```python
from build123d import *

# Parameters (mm, degrees)
F1_DEPTH = 2
F2_R     = 0.5
F3_R     = 2
F4_SIZE  = 0.49999


# Not quite as in the source:
# - a fillet or chamfer is up to 0.001 mm smaller than in the source, because OpenCascade refuses the exact size


with BuildPart() as f1:
    # F0 (on Top) → F1 (new body)
    with BuildSketch(Plane.XY):
        Polygon((-14.4337567297, 0), (-7.2168783649, 12.5), (7.2168783649, 12.5), (9.5262794416, 12.5), (10.68097998, 12.5), (17.8978583449, 0), (8.9489291724, -15.5), (-8.9489291724, -15.5), (-17.8978583449, 0), (-8.9489291724, 15.5), (8.9489291724, 15.5), (10.1036297108, 17.5), (-10.1036297108, 17.5), (-20.2072594216, 0), (-10.1036297108, -17.5), (10.1036297108, -17.5), (20.2072594216, 0), (11.8356805184, 14.5), (8.3715789032, 14.5), (-8.3715789032, 14.5), (-16.7431578065, 0), (-8.3715789032, -14.5), (8.3715789032, -14.5), (16.7431578065, 0), (14.4337567297, 0), (7.2168783649, -12.5), (-7.2168783649, -12.5), align=None)
    extrude(amount=F1_DEPTH)

    # F2
    f2_edges = [f1.edges().sort_by_distance(p)[0] for p in [
        (16.743158, 0, 1),
        (14.433757, 0, 1),
        (10.10363, 17.5, 1),
        (8.948929, 15.5, 1),
    ]]
    fillet(f2_edges, radius=F2_R)

    # F3
    f3_edges = [f1.edges().sort_by_distance(p)[0] for p in [
        (-10.10363, 17.5, 1),
        (-20.207259, 0, 1),
        (-10.10363, -17.5, 1),
        (10.10363, -17.5, 1),
        (20.207259, 0, 1),
        (11.835681, 14.5, 1),
        (-8.371579, 14.5, 1),
        (-16.743158, 0, 1),
        (-8.371579, -14.5, 1),
        (8.371579, -14.5, 1),
    ]]
    fillet(f3_edges, radius=F3_R)

    # F4 (size 0.5 in the source; OpenCascade refuses exactly that, so slightly less here)
    f4_edges = [f1.edges().sort_by_distance(p)[0] for p in [
        (12.629537, -7.125, 0),
        (8.216878, -14.232051, 0),
        (16.310145, -0.25, 0),
        (0, -14.5, 0),
        (15.299782, 0, 0),
        (-8.216878, -14.232051, 0),
        (14.472432, -0.066987, 0),
        (-12.557368, -7.25, 0),
        (10.753149, -6.375, 0),
        (-16.433757, 0, 0),
        (0, -12.5, 0),
        (-12.557368, 7.25, 0),
        (-10.825318, -6.25, 0),
        (-8.216878, 14.232051, 0),
        (-10.825318, 6.25, 0),
        (1.732051, 14.5, 0),
        (1.732051, 12.5, 0),
        (11.68098, 14.232051, 0),
        (14.289419, 6.25, 0),
        (16.02147, 7.25, 0),
        (13.423394, -7.75, 0),
        (19.897858, 0, 0),
        (0, -15.5, 0),
        (15.155445, -8.75, 0),
        (-13.423394, -7.75, 0),
        (9.948929, -17.232051, 0),
        (-13.423394, 7.75, 0),
        (0, -17.5, 0),
        (-0.144338, 15.5, 0),
        (-9.948929, -17.232051, 0),
        (8.910254, 15.566987, 0),
        (-15.155445, -8.75, 0),
        (9.381942, 16.25, 0),
        (-19.897858, 0, 0),
        (9.670617, 17.25, 0),
        (-15.155445, 8.75, 0),
        (0.144338, 17.5, 0),
        (-9.948929, 17.232051, 0),
        (12.629537, -7.125, 2),
        (8.216878, -14.232051, 2),
        (16.310145, -0.25, 2),
        (0, -14.5, 2),
        (15.299782, 0, 2),
        (-8.216878, -14.232051, 2),
        (14.472432, -0.066987, 2),
        (-12.557368, -7.25, 2),
        (10.753149, -6.375, 2),
        (-16.433757, 0, 2),
        (0, -12.5, 2),
        (-12.557368, 7.25, 2),
        (-10.825318, -6.25, 2),
        (-8.216878, 14.232051, 2),
        (-10.825318, 6.25, 2),
        (1.732051, 14.5, 2),
        (1.732051, 12.5, 2),
        (11.68098, 14.232051, 2),
        (14.289419, 6.25, 2),
        (16.02147, 7.25, 2),
        (13.423394, -7.75, 2),
        (19.897858, 0, 2),
        (0, -15.5, 2),
        (15.155445, -8.75, 2),
        (-13.423394, -7.75, 2),
        (9.948929, -17.232051, 2),
        (-13.423394, 7.75, 2),
        (0, -17.5, 2),
        (-0.144338, 15.5, 2),
        (-9.948929, -17.232051, 2),
        (8.910254, 15.566987, 2),
        (-15.155445, -8.75, 2),
        (9.381942, 16.25, 2),
        (-19.897858, 0, 2),
        (9.670617, 17.25, 2),
        (-15.155445, 8.75, 2),
        (0.144338, 17.5, 2),
        (-9.948929, 17.232051, 2),
    ]]
    chamfer(f4_edges, length=F4_SIZE)


solid = f1.part
```
Model file for the job. Use its own axes, mm. A direction names the side the tool comes from. Give positions to 0.01 mm unless a question says otherwise; leave off trailing zeros. Order: outer loops, then holes, each group sorted by start corner. A loop starts at its lowest first (then second) coordinate and runs counter-clockwise, first axis right, second up.
1) Mould opens along X. For faces 1 (the flat face through (-15, -8.52, 0.25)), 2 (the flat face through (16.072, 7.162, 0.993)), 3 (the conical face through (8.05, -13.97, 1.81)) say: +X half, -X half, draft (parallel to the pull), parting line (faces both ways), or undercut.
2) Wall check: probe 1 along Y at (x, z) = (1, 0.95); probe 2 along X at (y, z) = (11, 1.1); probe 3 along X at (y, z) = (11.5, 0.55). Give the ranges that are in metal, low to high.
3) Saw through at A-A, the plane x = 6. Count the separate pieces of the cut face and the enclosed holes in it, then the cut area to 3 significant figures.
4) Pin check, flat tips, straight feed: pin 1 (2 mm diameter, centred on x = -6.5, y = 9.5, fed in from +Z) (1 decimal); pin 2 (0.8 mm diameter, centred on x = 15, z = 1, fed in from +Y); pin 3 (1 mm diameter, centred on y = -4, z = 1, fed in from -X); pin 4 (1 mm diameter, centred on y = -7, z = 1.5, fed in from -X). Stop position of each tip, or through.
5) Saw through at D-D, the plane y = 6. Write the cut outline in (x, z), then the cut area to 3 significant figures.
6) Saw through at C-C, the plane x = 17. Write the cut outline in (y, z), then the cut area to 3 significant figures.
7) 3-axis set-ups, long thin cutter, end or side, ignore diameter. For faces 4 (the flat face through (9.378, 16.243, 0.993)), 5 (the flat face through (-13.36, -7.86, 0.99)), 6 (the flat face through (-13.572, -7.985, 0.253)), 7 (the flat face through (-14.879, 8.735, 0.253)), 8 (the flat face through (-13.708, 7.765, 1.754)): which of +Z, -Z, +X, -X, +Y, -Y reach the whole face in a straight line?
Computed:
1. face 1: -X half
1. face 2: +X half
1. face 3: undercut
2. probe 1: y = -17.5 to -15.5, -14.5 to -12.5, 12.5 to 14.5, 15.5 to 17.5
2. probe 2: x = -13.86 to -11.55, -10.39 to -8.08, 11.55 to 13.86
2. probe 3: x = -13.57 to -11.26, -10.1 to -7.79, 11.26 to 13.57
3. separate pieces: 4
3. enclosed holes: 0
3. area: 14.0 mm2
4. pin 1: passes through
4. pin 2: stops at y = 9.71
4. pin 3: stops at x = -18.19
4. pin 4: stops at x = -16.45
5. outline: (-16.74, 0.5) - (-16.17, 0) - (-15.01, 0) - (-14.43, 0.5) - (-14.43, 1.5) - (-15.01, 2) - (-16.17, 2) - (-16.74, 1.5) - close; (-13.28, 0.5) - (-12.7, 0) - (-11.55, 0) - (-10.97, 0.5) - (-10.97, 1.5) - (-11.55, 2) - (-12.7, 2) - (-13.28, 1.5) - close; (14.43, 0.5) - (15.01, 0) - (16.17, 0) - (16.74, 0.5) - (16.74, 1.5) - (16.17, 2) - (15.01, 2) - (14.43, 1.5) - close
5. area: 12.1 mm2
6. outline: (-5.56, 0.5) - (-4.56, 0) - (-2.56, 0) - (-1.56, 0.5) - (-1.56, 1.5) - (-2.56, 2) - (-4.56, 2) - (-5.56, 1.5) - close; (1.56, 0.5) - (2.56, 0) - (4.56, 0) - (5.56, 0.5) - (5.56, 1.5) - (4.56, 2) - (2.56, 2) - (1.56, 1.5) - close
6. area: 14.0 mm2
7. face 4: +Z, -Z, +X
7. face 5: +Z, -Z
7. face 6: -Z
7. face 7: -Z, -X, +Y
7. face 8: +Z
